from build123d import *

# Parameters (mm, degrees)
SKETCH1_R           = 1.25
BOSS_EXTRUDE1_DEPTH = 3
FILLET1_R           = 3
SKETCH2_R           = 3
SKETCH2_R_2         = 1.25
BOSS_EXTRUDE2_DEPTH = 7
SKETCH4_R           = 2.125
CUT_EXTRUDE1_DEPTH  = 11


with BuildPart() as part:
    # Sketch1 → Boss-Extrude1 (new body)
    with BuildSketch(Plane(origin=(0, 0, 0), x_dir=(1, 0, 0), z_dir=(0, 1, 0))):
        Polygon((0, 0), (110, 0), (110, 16), (110, 100), (0, 100), (0, 16), align=None)
        with Locations((4, 96)):
            Circle(SKETCH1_R, mode=Mode.SUBTRACT)
        with Locations((106, 96)):
            Circle(SKETCH1_R, mode=Mode.SUBTRACT)
        with Locations((106, 20)):
            Circle(SKETCH1_R, mode=Mode.SUBTRACT)
        with Locations((4, 20)):
            Circle(SKETCH1_R, mode=Mode.SUBTRACT)
    extrude(amount=BOSS_EXTRUDE1_DEPTH)

    # Fillet1
    fillet1_edges = [part.edges().sort_by_distance(p)[0] for p in [
        (0, 1.5, -100),
        (110, 1.5, -100),
        (110, 1.5, 0),
        (0, 1.5, 0),
    ]]
    fillet(fillet1_edges, radius=FILLET1_R)

    # Sketch2 → Boss-Extrude2 (add)
    with BuildSketch(Plane(origin=(0, 3, 0), x_dir=(1, 0, 0), z_dir=(0, 1, 0))):
        with Locations((4, 96)):
            Circle(SKETCH2_R)
        with Locations((4, 96)):
            Circle(SKETCH2_R_2, mode=Mode.SUBTRACT)
        with Locations((106, 96)):
            Circle(SKETCH2_R)
        with Locations((106, 96)):
            Circle(SKETCH2_R_2, mode=Mode.SUBTRACT)
        with Locations((106, 20)):
            Circle(SKETCH2_R)
        with Locations((106, 20)):
            Circle(SKETCH2_R_2, mode=Mode.SUBTRACT)
        with Locations((4, 20)):
            Circle(SKETCH2_R)
        with Locations((4, 20)):
            Circle(SKETCH2_R_2, mode=Mode.SUBTRACT)
    extrude(amount=BOSS_EXTRUDE2_DEPTH)

    # Sketch4 → Cut-Extrude1 (cut, through all)
    with BuildSketch(Plane.XZ):
        with Locations((10, -6)):
            Circle(SKETCH4_R)
        with Locations((100, -6)):
            Circle(SKETCH4_R)
    extrude(amount=-CUT_EXTRUDE1_DEPTH, mode=Mode.SUBTRACT)


solid = part.part
Read the model definition and answer for the solid it produces. Units are mm, in the model's axes. A direction names the side the tool comes from. Coordinates: 2 decimals unless noted, no trailing zeros. Loops run counter-clockwise (first coordinate to the right, second up) from the corner with the lowest first, then second, coordinate; pieces in that order, holes last.
Q1. Which of the six approach directions +Z, -Z, +X, -X, +Y, -Y give full straight-line access (tool end or side, diameter ignored) to faces 4 (the face through (110, 1, -49)), 5 (the face through (3.35, 6.45, -93.07))?
Q2. The mould has two halves that part along X. Classify faces 1 (the face through (109.14, 1.52, -99.1)), 2 (the face through (107, 10, -95)), 3 (the face through (107.155, 4.93, -19.521)): +X half, -X half, draft (parallel to the pull), parting line (faces both ways), or undercut.
Q3. The part is cut by section A-A on x = 100. Write down the section's boundary in (y, z) (3 decimals), and give its area (3 significant figures).
Q4. Consider probe 1 along X at (y, z) = (5.5, -96); probe 2 along Z at (x, y) = (106, 4.75); probe 3 along Z at (x, y) = (10, 0.95) (3 decimals). Determine where each line is inside the solid, lowest interval first.
Q5. The part is cut by section B-B on y = 4.5. Write down the section's boundary in (x, z), and give its area (3 significant figures).
Q6. This flat-tipped pin is pushed along its axis until it touches: pin 1 Ø1 at (x, z) = (40, -17.5) entering from +Y. Where does it stop, or does it pass through?
Q7. The part is cut by section D-D on z = -36.5. Write down the section's boundary in (x, y).
Q8. The part is cut by section C-C on z = -20. Write down the section's boundary in (x, y).
Results below:
1. face 4: +Z, -Z, +X, +Y, -Y
1. face 5: +Y
2. face 1: +X half
2. face 2: draft
2. face 3: undercut
3. outline: (0, -100) - (3, -100) - (3, -8.125) - (0, -8.125) - close; (0, -3.875) - (3, -3.875) - (3, 0) - (0, 0) - close
3. area: 287 mm2
4. probe 1: x = 1 to 2.75, 5.25 to 7, 103 to 104.75, 107.25 to 109
4. probe 2: z = -99 to -97.25, -94.75 to -93, -23 to -21.25, -18.75 to -17
4. probe 3: z = -100 to -8.125, -3.875 to 0
5. outline: circle Ø6 at (4, -96); circle Ø6 at (4, -20); circle Ø6 at (106, -96); circle Ø6 at (106, -20); hole circle Ø2.5 at (4, -96); hole circle Ø2.5 at (4, -20); hole circle Ø2.5 at (106, -96); hole circle Ø2.5 at (106, -20)
5. area: 93.5 mm2
6. pin 1: stops at y = 3
7. outline: (0, 0) - (110, 0) - (110, 3) - (0, 3) - close
8. outline: (0, 0) - (2.75, 0) - (2.75, 10) - (1, 10) - (1, 3) - (0, 3) - close; (5.25, 0) - (104.75, 0) - (104.75, 10) - (103, 10) - (103, 3) - (7, 3) - (7, 10) - (5.25, 10) - close; (107.25, 0) - (110, 0) - (110, 3) - (109, 3) - (109, 10) - (107.25, 10) - close
